from build123d import *

# Parameters (mm, degrees)
SKETCH_4_W          = 400
SKETCH_4_H          = 250
EXTRUDE_4_DEPTH     = 200
SKETCH_10_R         = 25
CUT_EXTRUDE_1_DEPTH = 180
FILLET_3_R          = 15
SKETCH_9_R          = 125
EXTRUDE_8_DEPTH     = 250
FILLET_4_R          = 25
SKETCH_5_R          = 150
SKETCH_5_R_2        = 100
EXTRUDE_5_DEPTH     = 15
SKETCH_6_R          = 115
SKETCH_6_R_2        = 100
EXTRUDE_6_DEPTH     = 6
SKETCH_13_R         = 6
CUT_EXTRUDE_2_DEPTH = 15


with BuildPart() as part:
    # 草图4 → 凸台-拉伸4 (new body)
    with BuildSketch(Plane(origin=(0, 0, 0), x_dir=(0, 0, -1), z_dir=(1, 0, 0))):
        Rectangle(SKETCH_4_W, SKETCH_4_H)
    extrude(amount=-EXTRUDE_4_DEPTH)

    # 草图10 → 切除-拉伸1 (cut)
    with BuildSketch(Plane(origin=(0, 0, 0), x_dir=(0, 0, -1), z_dir=(1, 0, 0))):
        Circle(SKETCH_10_R)
    extrude(amount=-CUT_EXTRUDE_1_DEPTH, mode=Mode.SUBTRACT)

    # 圆角3
    fillet_3_edges = [part.edges().sort_by_distance(p)[0] for p in [
        (-200, 0, -200),
        (-200, 125, 0),
        (-200, 0, 200),
        (0, 125, 0),
        (0, 0, -200),
        (0, -125, 0),
        (0, 0, 200),
        (-200, -125, 0),
        (-100, 125, 200),
        (-100, 125, -200),
        (-100, -125, -200),
        (-100, -125, 200),
    ]]
    fillet(fillet_3_edges, radius=FILLET_3_R)

    # 草图9 → 凸台-拉伸8 (add)
    with BuildSketch(Plane.XY.offset(200)):
        with Locations(Location((-100, 0, 0), (0, 0, 132.843643044))):
            Circle(SKETCH_9_R)
    extrude(amount=EXTRUDE_8_DEPTH)

    # 圆角4
    fillet_4_edges = [part.edges().sort_by_distance(p)[0] for p in [
        (-14.999999999, -91.651513899, 450),
    ]]
    fillet(fillet_4_edges, radius=FILLET_4_R)

    # 草图12 → 旋转1 (revolve)
    with BuildSketch(Plane.XY, mode=Mode.PRIVATE) as revolve_1_sk:
        Polygon((0, 75), (50, 125), (50, 110.857864376), (0, 60.857864376), align=None)
    revolve(revolve_1_sk.sketch.rotate(Axis((-1000, 0, 0), (1, 0, 0)), 90), axis=Axis((-1000, 0, 0), (1, 0, 0)))

    # 草图5 → 凸台-拉伸5 (add)
    with BuildSketch(Plane(origin=(50, 0, 0), x_dir=(0, 0, -1), z_dir=(1, 0, 0))):
        Circle(SKETCH_5_R)
        Circle(SKETCH_5_R_2, mode=Mode.SUBTRACT)
    extrude(amount=EXTRUDE_5_DEPTH)

    # 草图6 → 凸台-拉伸6 (add)
    with BuildSketch(Plane(origin=(65, 0, 0), x_dir=(0, 0, -1), z_dir=(1, 0, 0))):
        Circle(SKETCH_6_R)
        Circle(SKETCH_6_R_2, mode=Mode.SUBTRACT)
    extrude(amount=EXTRUDE_6_DEPTH)

    # 草图13 → 切除-拉伸2 (cut)
    with BuildSketch(Plane(origin=(65, 0, 0), x_dir=(0, 0, -1), z_dir=(1, 0, 0))):
        with Locations((93.691648507, 93.691648507)):
            Circle(SKETCH_13_R)
        with Locations((-93.691648507, -93.691648507)):
            Circle(SKETCH_13_R)
        with Locations((-93.691648507, 93.691648507)):
            Circle(SKETCH_13_R)
        with Locations((93.691648507, -93.691648507)):
            Circle(SKETCH_13_R)
    extrude(amount=-CUT_EXTRUDE_2_DEPTH, mode=Mode.SUBTRACT)


solid = part.part
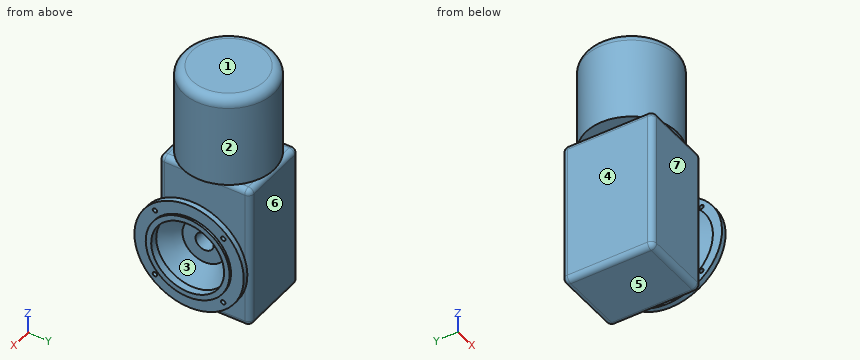
The listing builds one solid part. Answer for the finished solid, in the listing's coordinates (mm). Face numbers are marked on the shaded views. A direction names the side the tool comes from. Give positions to 0.01 mm unless a question says otherwise; leave off trailing zeros. Write each loop counter-clockwise with the first axis right and the second up, starting at its lowest first coordinate (ties: lowest second). Pieces come first, ordered by that corner, then holes.
1) Section D-D (z = 283) is taken. Write down the section's boundary in (x, y).
2) For a pull along Z with two mould halves and no side action, classify the marked faces 1, 2 and 3 as pulls with the +Z half, pulls with the -Z half, needs draft (parallel to the pull), parting line crosses it, or undercut.
3) Find the intervals of material crossed by L1, parallel to Z at x = 11, y = -46; L2, parallel to X at y = -31, z = -141.5; L3, parallel to Y at x = -46, z = 98, in increasing order.
4) Section A-A (x = -100) is taken. Write down the section's boundary in (y, z).
5) Section C-C (z = 143) is taken. Write down the section's boundary in (x, y), and give its area (3 significant figures).
6) Given P1, Ø6, axis at x = -92, y = 107.5, coming from the +Z side; P2, Ø4, axis at y = 58.5, z = -20.5, coming from the +X side; P3, Ø3, axis at y = -5, z = -88.5, coming from the -X side; P4, Ø16.5, axis at x = -126.5, y = 115, coming from the -Z side, each flat-ended and moving along its own axis, determine where each tip first touches the part or whether it passes through.
7) A tool of negligible diameter and unlimited length cuts with its end or side. For the marked faces 4, 5, 6 and 7, from which of +Z, -Z, +X, -X, +Y, -Y can it reach the whole face along a straight path? Write none if from no direction.
Response:
1. outline: circle Ø250 at (-100, 0)
2. face 1: pulls with the +Z half
2. face 2: needs draft
2. face 3: undercut
3. L1: z = -72.66 to -55.2, 55.2 to 72.66, 200 to 439.79
3. L2: x = -200 to 0, 50 to 65
3. L3: y = -125 to 125
4. outline: (-125, -185) arc R15 ccw to (-110, -200) - (110, -200) arc R15 ccw to (125, -185) - (125, 185) arc R15 ccw to (110, 200) - (125, 200) - (125, 425) arc R25 ccw to (100, 450) - (-100, 450) arc R25 ccw to (-125, 425) - (-125, 200) - (-110, 200) arc R15 ccw to (-125, 185) - close; hole circle Ø50 at (0, 0)
5. outline: (-200, -110) arc R15 ccw to (-185, -125) - (-15, -125) arc R15 ccw to (0, -110) - (0, 110) arc R15 ccw to (-15, 125) - (-185, 125) arc R15 ccw to (-200, 110) - close; (50, -45.29) - (65, -45.29) - (65, 45.29) - (50, 45.29) - close
5. area: 51,200 mm2
6. P1: stops at z = 449.54
6. P2: stops at x = 3.13
6. P3: stops at x = -200
6. P4: stops at z = -200
7. face 4: -Z, -X, +Y, -Y
7. face 5: -Z, +X, -X, +Y, -Y
7. face 6: +Z, -Z, -X, +Y
7. face 7: +Z, -Z, -X, -Y
